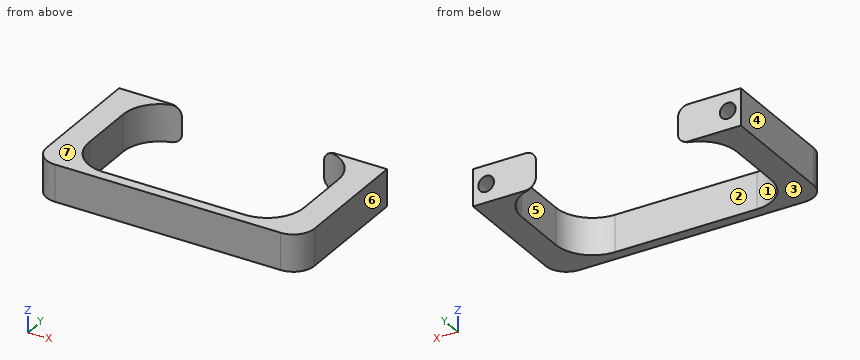
Autodesk Inventor part; units mm, degrees
ref_plane "YZ Plane" through (0, 0, 0) normal (1, 0, 0) x (0, 1, 0)
ref_plane "XZ Plane" through (0, 0, 0) normal (0, 1, 0) x (-1, 0, 0)
ref_plane "XY Plane" through (0, 0, 0) normal (0, 0, 1) x (1, 0, 0)
sketch "Sketch1" plane through (0, 0, 0) normal (0, 0, 1) x (1, 0, 0)
  line L0 (17, -8.875) -> (-17, -8.875) construction
  line L1 (-17, -8.875) -> (-17, 8.875) construction
  line L2 (-17, 8.875) -> (17, 8.875) construction
  line L3 (17, 8.875) -> (17, -8.875) construction
  line L4 (17, -8.875) -> (-17, 8.875) construction
  line L5 (-17, -8.875) -> (17, 8.875) construction
  line L6 (20.5, 12.375) -> (-20.5, 12.375)
  line L7 (-20.5, 12.375) -> (-20.5, -12.375)
  line L8 (-20.5, -12.375) -> (20.5, -12.375)
  line L9 (20.5, -12.375) -> (20.5, 12.375)
  line L10 (20.5, 12.375) -> (-20.5, -12.375) construction
  line L11 (-20.5, 12.375) -> (20.5, -12.375) construction
  line L12 (-25.5, -14.375) -> (25.5, -14.375)
  line L13 (25.5, -14.375) -> (25.5, 14.375)
  line L14 (25.5, 14.375) -> (-25.5, 14.375)
  line L15 (-25.5, 14.375) -> (-25.5, -14.375)
  line L16 (-25.5, -14.375) -> (25.5, 14.375) construction
  line L17 (25.5, -14.375) -> (-25.5, 14.375) construction
  line L18 (-20.5, 12.375) -> (-25.5, 12.375)
  line L19 (20.5, 12.375) -> (25.5, 12.375)
  point P0 (0, 0)
  dimension "d0" = 34
  dimension "d1" = 17.75
  dimension "d2" = 41
  dimension "d3" = 24.75
  dimension "d4" = 51
  dimension "d5" = 28.75
extrude "Extrusion1" add sketch "Sketch1" along normal blind 7 contours L19 L13 L12 L15 L18 L7 L8 L9
sketch "Sketch3" plane through (-25.5, 12.375, 0) normal (0, 1, 0) x (1, 0, 0)
  line L0 (0, 0) -> (0, -7) construction
  line L1 (0, -3.5) -> (2.5, -3.5) construction
  line L2 (51, 0) -> (51, -7) construction
  line L3 (51, -3.5) -> (48.5, -3.5) construction
  circle A0 centre (2.5, -3.5) radius 1.5
  circle A1 centre (48.5, -3.5) radius 1.5
  point P0 (25.5, 0)
  dimension "d18" = 2.5
  dimension "d19" = 2.5
  dimension "d20" = 3
  dimension "d21" = 3
extrude "Extrusion3" cut sketch "Sketch3" against normal blind 7
fillet "Fillet1" radius 7 2 edges at (-20.5, -12.375, 3.5) (20.5, -12.375, 3.5)
fillet "Fillet2" radius 4 2 edges at (-25.5, -14.375, 3.5) (25.5, -14.375, 3.5)
sketch "Sketch4" plane through (0, 0, 7) normal (0, 0, 1) x (1, 0, 0)
  line L0 (-20.5, 12.375) -> (-25.5, 12.375) construction
  line L1 (-20.5, 12.375) -> (-20.5, 10.375) construction
  line L2 (-20.5, -5.375) -> (-20.5, 12.375) construction
  line L3 (-20.5, 12.375) -> (-18.5, 12.375) construction
  line L4 (-18.5, 12.375) -> (-16.5, 12.375) construction
  line L5 (-20.5, 10.375) -> (-13.5, 10.375) construction
  line L6 (-13.5, 12.375) -> (-13.5, 5.375) construction
  circle A0 centre (-13.5, 5.375) radius 7
  line L7 (-20.5, 12.375) -> (-13.5, 12.375)
  line L8 (-20.5, 5.375) -> (-20.5, 12.375)
  point P0 (0, 0)
  dimension "d27" = 2
  dimension "d28" = 90
  dimension "d31" = 7
  dimension "d32" = 7
  dimension "d33" = 7
extrude "Extrusion4" add sketch "Sketch4" against normal up to surface (7 mm away) contours A0 L8 L7
mirror "Mirror1" about plane through (0, 0, 0) normal (1, 0, 0) of "Extrusion4"
sketch "Sketch5" plane through (-25.5, 12.375, 7) normal (0, 1, 0) x (1, 0, 0)
  line L0 (0, 7) -> (0, 0) construction
  line L1 (12, 0) -> (0, 0) construction
  line L2 (0, 7) -> (10, 7) construction
  line L3 (12, 5) -> (12, 2) construction
  line L4 (10, 0) -> (0, 0) construction
  line L5 (0, 0) -> (0, 7) construction
  arc A0 (12, 5) -> (10, 7) centre (10, 5) ccw
  arc A1 (10, 0) -> (12, 2) centre (10, 2) ccw
  line L6 (12, 5) -> (12, 2)
  line L7 (10, 0) -> (0, 0)
  line L8 (0, 7) -> (0, 0)
  line L9 (0, 7) -> (10, 7)
  line L10 (39, 7) -> (39, 0) construction
  line L11 (51, 0) -> (39, 0) construction
  line L12 (41, 7) -> (51, 7) construction
  line L13 (51, 7) -> (51, 0) construction
  line L14 (51, 0) -> (41, 0) construction
  line L15 (39, 2) -> (39, 5) construction
  arc A2 (41, 7) -> (39, 5) centre (41, 5) ccw
  arc A3 (39, 2) -> (41, 0) centre (41, 2) ccw
  line L16 (41, 7) -> (51, 7)
  line L17 (51, 0) -> (51, 7)
  line L18 (51, 0) -> (41, 0)
  line L19 (39, 2) -> (39, 5)
  line L20 (12, 0) -> (12, 7)
  line L21 (10, 7) -> (12, 7)
  line L22 (12, 7) -> (12, 5)
  line L23 (12, 2) -> (12, 0)
  line L24 (12, 0) -> (10, 0)
  line L25 (41, 7) -> (39, 7)
  line L26 (39, 5) -> (39, 7)
  line L27 (39, 2) -> (39, 0)
  line L28 (41, 0) -> (39, 0)
  point P0 (25.5, 7)
  dimension "d36" = 2
  dimension "d37" = 2
  dimension "d38" = 2
extrude "Extrusion5" cut sketch "Sketch5" against normal blind 1 contours A0 L21 L20 | L20 L24 A1 | A2 L26 L25 | A3 L28 L27
properties part number "Clamp_v4_bot"
Here's how the part is built. I have some questions about the finished solid (model axes, mm). Face numbers are marked on the shaded views. A direction names the side the tool comes from. Round coordinates to 2 decimals unless told otherwise and drop trailing zeros. Order: outer loops, then holes, each group sorted by start corner. A loop starts at its lowest first (then second) coordinate and runs counter-clockwise, first axis right, second up. Notation, with made-up numbers: M 81,59 L 108,59 A26 ccw 108,73 Z; hole C 81,23 d9. An arc over 180 degrees is marked long. Answer in a Markdown table with one row per item.
Item 1: If I drill on L1, parallel to X at y = 10.5, z = 3.5; L2, parallel to X at y = 8.5, z = 3.5; L3, parallel to Z at x = -23, y = 8.75, over which ranges is the centre line in solid material (lowest first)? Write a range as from..to.
A:
| item | result |
|---|---|
| L1 | x = -25.5..-24.5, -21.5..-18.27, 18.27..21.5, 24.5..25.5 |
| L2 | x = -25.5..-24.5, -21.5..-19.76, 19.76..21.5, 24.5..25.5 |
| L3 | z = 0..2, 5..7 |
Item 2: Imagine slicing it at D-D, the plane x = 23. Write out the boundary of the cut face in (y, z) (3 decimals).
A:
| item | result |
|---|---|
| outline | M -14.083,0 L 12.375,0 L 12.375,2 L 5.375,2 L 5.375,5 L 12.375,5 L 12.375,7 L -14.083,7 Z |
Item 3: Imagine slicing it at C-C, the plane z = 3.5. Write out the boundary of the cut face in (x, y) (3 decimals).
A:
| item | result |
|---|---|
| outline | M -25.5,-10.375 A4 ccw -21.5,-14.375 L 21.5,-14.375 A4 ccw 25.5,-10.375 L 25.5,12.375 L 24.5,12.375 L 24.5,5.375 L 21.5,5.375 L 21.5,12.375 L 13.5,12.375 A7 cw 20.5,5.375 L 20.5,-5.375 A7 cw 13.5,-12.375 L -13.5,-12.375 A7 cw -20.5,-5.375 L -20.5,5.375 A7 cw -13.5,12.375 L -21.5,12.375 L -21.5,5.375 L -24.5,5.375 L -24.5,12.375 L -25.5,12.375 Z |
Item 4: Imagine slicing it at A-A, the plane y = -1.25. Write out the boundary of the cut face in (x, z), and give its area (3 significant figures).
A:
| item | result |
|---|---|
| outline | M -25.5,0 L -20.5,0 L -20.5,7 L -25.5,7 Z; M 20.5,0 L 25.5,0 L 25.5,7 L 20.5,7 Z |
| area | 70.0 mm2 |
Item 5: For the marked faces 1, 2 and 3, which set-ups out of +Z, -Z, +X, -X, +Y, -Y let a thin tool reach every point of the face, with its end or its side?
A:
| item | result |
|---|---|
| face 1 | +Z, -Z |
| face 2 | +Z, -Z, +Y |
| face 3 | -Z, +X, -X, +Y, -Y |
Item 6: Imagine slicing it at B-B, the plane x = 17. Write out the boundary of the cut face in (y, z) (3 decimals).
A:
| item | result |
|---|---|
| outline | M -14.375,0 L -11.437,0 L -11.437,7 L -14.375,7 Z; M 11.437,0 L 12.375,0 L 12.375,7 L 11.437,7 Z |
Item 7: I'm going to push flat-ended pins straight in: pin 1 (0.9 mm diameter, centred on x = 22.5, z = 3, fed in from +Y) (3 decimals); pin 2 (4 mm diameter, centred on x = -23, z = 3.5, fed in from +Y) (3 decimals); pin 3 (2.5 mm diameter, centred on x = 23, z = 3.5, fed in from -Y). Where does each tip first touch, or does it pass through?
A:
| item | result |
|---|---|
| pin 1 | stops at y = 5.375 |
| pin 2 | stops at y = 12.375 |
| pin 3 | stops at y = -14.37 |
Item 8: Thinking about a two-plate mould opening in X: for the marked faces 4, 5, 6 and 7, which applies, +X half, -X half, draft (parallel to the pull), parting line (faces both ways), or undercut?
A:
| item | result |
|---|---|
| face 4 | -X half |
| face 5 | undercut |
| face 6 | +X half |
| face 7 | draft |
